Geometry check sheet. Reference: drawing and pictorial views, mm from the part's lowest x, y, z. Give positions to 0.01 mm unless a question says otherwise; leave off trailing zeros. Order: outer loops, then holes, each group sorted by start corner. A loop starts at its lowest first (then second) coordinate and runs counter-clockwise, first axis right, second up.
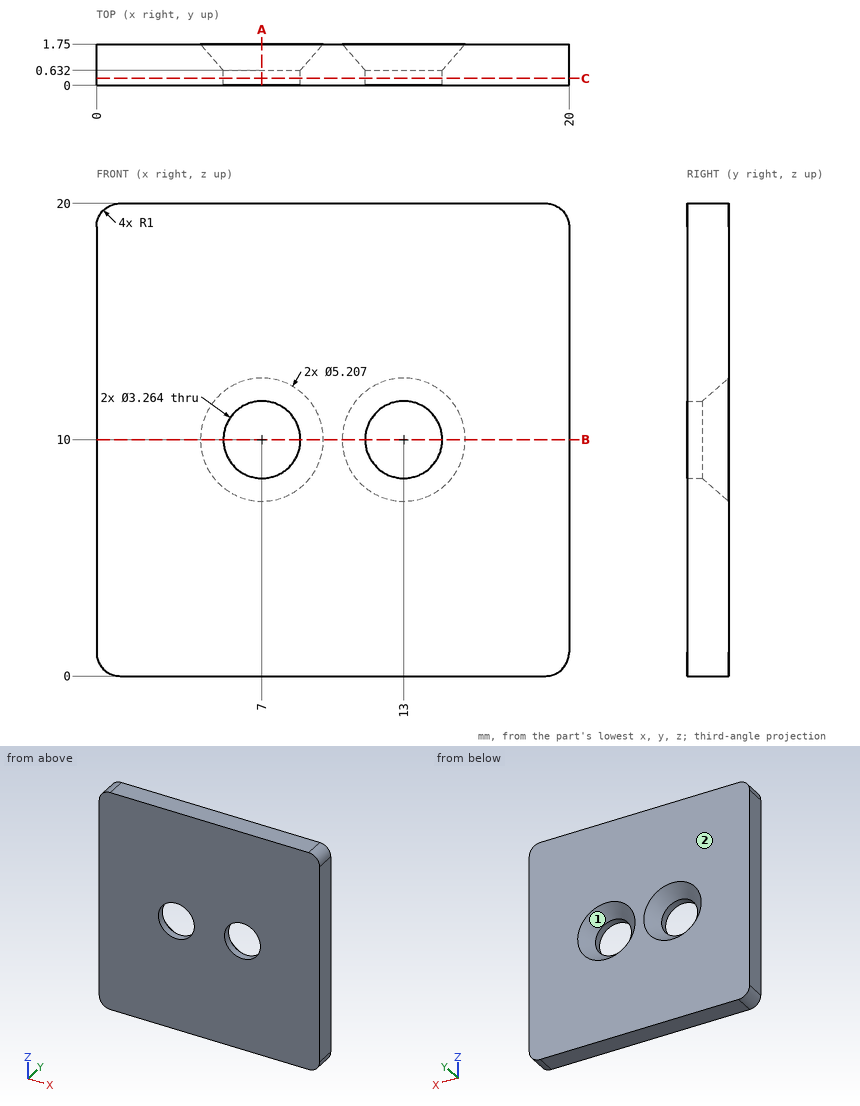
1) Material ranges on L1, parallel to X at y = 0.5, z = 10; L2, parallel to Z at x = 13, y = 0.25; L3, parallel to X at y = 1.35, z = 8 (1 decimal), recorded low to high.
Recorded:
L1: x = 0 to 5.37, 8.63 to 11.37, 14.63 to 20
L2: z = 0 to 8.37, 11.63 to 20
L3: x = 0 to 6, 8 to 12, 14 to 20
2) Section check A-A, the plane x = 7. Record the cut outline in (y, z).
Recorded:
outline: (0, 0) - (1.75, 0) - (1.75, 7.4) - (0.63, 8.37) - (0, 8.37) - close; (0, 11.63) - (0.63, 11.63) - (1.75, 12.6) - (1.75, 20) - (0, 20) - close
3) Draft check along X on the marked faces 1 and 2. Enter one of: +X half, -X half, draft (parallel to the pull), parting line (faces both ways), or undercut.
Recorded:
face 1: undercut
face 2: draft
4) Section check C-C, the plane y = 0.3. Record the cut outline in (x, z), then the cut area to 3 significant figures.
Recorded:
outline: (0, 1) arc R1 ccw to (1, 0) - (19, 0) arc R1 ccw to (20, 1) - (20, 19) arc R1 ccw to (19, 20) - (1, 20) arc R1 ccw to (0, 19) - close; hole circle Ø3.26 at (7, 10); hole circle Ø3.26 at (13, 10)
area: 382 mm2
5) Depth check by flat-ended pin: pin 1 Ø4 at (x, z) = (7, 10) entering from +Y (1 decimal); pin 2 Ø3 at (x, z) = (9.5, 6.5) entering from -Y. Enter the tip coordinate at first touch or a pass-through.
Recorded:
pin 1: stops at y = 1.1
pin 2: stops at y = 0
6) Section check B-B, the plane z = 10. Record the cut outline in (x, y), then the cut area to 3 significant figures.
Recorded:
outline: (0, 0) - (5.37, 0) - (5.37, 0.63) - (4.4, 1.75) - (0, 1.75) - close; (8.63, 0) - (11.37, 0) - (11.37, 0.63) - (10.4, 1.75) - (9.6, 1.75) - (8.63, 0.63) - close; (14.63, 0) - (20, 0) - (20, 1.75) - (15.6, 1.75) - (14.63, 0.63) - close
area: 21.4 mm2
